Source: CAD feature listing. Evaluate the final solid. Frame: model axes, mm. Face numbers are marked on the shaded views. A direction names the side the tool comes from. Give positions to 0.01 mm unless a question says otherwise; leave off trailing zeros. Write each loop counter-clockwise with the first axis right and the second up, starting at its lowest first coordinate (ties: lowest second). Pieces come first, ordered by that corner, then holes. Notation, with made-up numbers: (34, 48.5) - (58, 48.5) arc R21 ccw to (58, 72.5) - close; hole circle Ø6 at (75.25, -4.75). An arc over 180 degrees is marked (long way). One line per question, with ' | ' between items. Start each with the question number.
(1) Section B-B, the plane y = 9. Return loops of the section in (x, z).
(2) Section D-D, the plane y = 0. Return loops of the section in (x, z), plus the area to 3 significant figures.
(3) Ray query, line 1 (Z direction, x = 8.75, y = 6); line 2 (Z direction, x = -1.5, y = -5); line 3 (Y direction, x = 5.75, z = 2). Return the intervals inside material, ascending. Write a range as [from, to].
(4) Access query for the marked faces 1, 2 and 3. Directions: +Z, -Z, +X, -X, +Y, -Y. A direction counts if a zero-diameter tool reaches every point of the face in a straight line with its end or side. Return the directions, or none.
(5) Pin query (flat end, axial travel): pin 1 (5 mm diameter, centred on x = -3, z = 7, fed in from -Y); pin 2 (1.5 mm diameter, centred on x = -3, z = 7.5, fed in from -Y); pin 3 (3.5 mm diameter, centred on x = -7.79, y = -4.5, fed in from +Z). Return the tip coordinate at first contact, or that it passes through.
(6) Section C-C, the plane y = -4.5. Return loops of the section in (x, z).
(7) Section A-A, the plane x = 0. Return loops of the section in (y, z), plus the area to 3 significant figures.
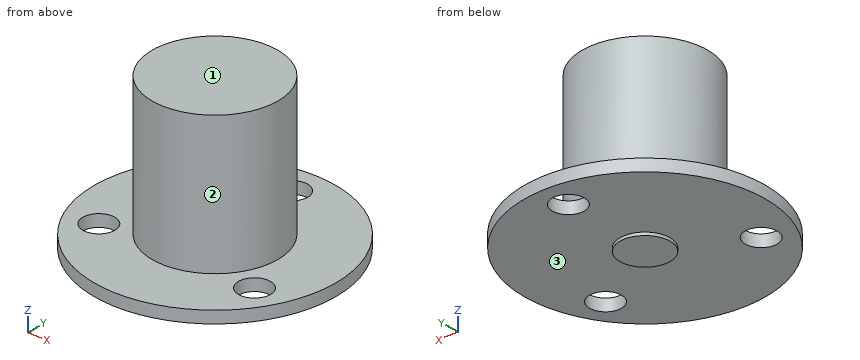
Autodesk Inventor part; units mm, degrees
ref_plane "YZ Plane" through (0, 0, 0) normal (1, 0, 0) x (0, 1, 0)
ref_plane "XZ Plane" through (0, 0, 0) normal (0, 1, 0) x (-1, 0, 0)
ref_plane "XY Plane" through (0, 0, 0) normal (0, 0, 1) x (1, 0, 0)
sketch "Náčrt1" plane through (0, 0, 0) normal (0, 0, 1) x (1, 0, 0)
  circle A0 centre (0, 0) radius 12
  dimension "d0" = 24
extrude "Vysunutí1" add sketch "Náčrt1" along normal blind 1.2
sketch "Náčrt2" plane through (0, 0, 1.2) normal (0, 0, 1) x (1, 0, 0)
  circle A0 centre (0, 0) radius 9 construction
  circle A1 centre (0, 9) radius 1.6
  circle A2 centre (-7.7942, -4.5) radius 1.6
  circle A3 centre (7.7942, -4.5) radius 1.6
  dimension "d3" = 18
  dimension "d4" = 3.2
  dimension "d7" = 360
extrude "Vysunutí2" cut sketch "Náčrt2" against normal through all
sketch "Náčrt3" plane through (0, 0, 1.2) normal (0, 0, 1) x (1, 0, 0)
  circle A0 centre (0, 0) radius 6.25
  dimension "d11" = 12.5
extrude "Vysunutí3" add sketch "Náčrt3" along normal blind 13.8
sketch "Náčrt4" plane through (0, 0, 0) normal (0, 0, -1) x (-1, 0, 0)
  circle A0 centre (0, 0) radius 2.5
  dimension "d14" = 5
extrude "Vysunutí4" add sketch "Náčrt4" along normal blind 0.3
properties part number "OtocnaKontaktniPruchodka"
Check sheet entries:
1) outline: (-7.94, 0) - (-1.6, 0) - (-1.6, 1.2) - (-7.94, 1.2) - close; (1.6, 0) - (7.94, 0) - (7.94, 1.2) - (1.6, 1.2) - close
2) outline: (-12, 0) - (-2.5, 0) - (-2.5, -0.3) - (2.5, -0.3) - (2.5, 0) - (12, 0) - (12, 1.2) - (6.25, 1.2) - (6.25, 15) - (-6.25, 15) - (-6.25, 1.2) - (-12, 1.2) - close | area: 203 mm²
3) line 1: [0, 1.2] | line 2: [0, 15] | line 3: [-2.45, 2.45]
4) face 1: +Z, +X, -X, +Y, -Y | face 2: +Z | face 3: -Z
5) pin 1: y = -6.23 | pin 2: y = -5.83 | pin 3: z = 1.2
6) outline: (-11.12, 0) - (-9.39, 0) - (-9.39, 1.2) - (-11.12, 1.2) - close; (-6.19, 0) - (6.19, 0) - (6.19, 1.2) - (4.34, 1.2) - (4.34, 15) - (-4.34, 15) - (-4.34, 1.2) - (-6.19, 1.2) - close; (9.39, 0) - (11.12, 0) - (11.12, 1.2) - (9.39, 1.2) - close
7) outline: (-12, 0) - (-2.5, 0) - (-2.5, -0.3) - (2.5, -0.3) - (2.5, 0) - (7.4, 0) - (7.4, 1.2) - (6.25, 1.2) - (6.25, 15) - (-6.25, 15) - (-6.25, 1.2) - (-12, 1.2) - close; (10.6, 0) - (12, 0) - (12, 1.2) - (10.6, 1.2) - close | area: 199 mm²
